Geometry: final body of the model. Coordinates: model frame, mm. A direction names the side the tool comes from. Give positions to 0.01 mm unless a question says otherwise; leave off trailing zeros. Loops run counter-clockwise (first coordinate to the right, second up) from the corner with the lowest first, then second, coordinate; pieces in that order, holes last. Notation, with made-up numbers: (5.5, 9) - (25.5, 9) arc R8 ccw to (25.5, 16) - close; hole circle Ø2 at (35, -18.5). An arc over 180 degrees is marked (long way). Use one line per item in the form item = value.
```python
from build123d import *

# Parameters (mm, degrees)
F1_DEPTH = 100
F2_T     = -2
F3_R     = 40
F4_DEPTH = 2
F5_R     = 4
F6_DEPTH = 2
F5_R_2   = 5
F7_DEPTH = 10
F8_SIZE2 = 3
F8_SIZE  = 0.6


with BuildPart() as f1:
    # F0 (on Front) → F1 (new body)
    with BuildSketch(Plane.XZ):
        Polygon((34.6410161514, -60), (69.2820323028, 0), (34.6410161514, 60), (-34.6410161514, 60), (-69.2820323028, 0), (-34.6410161514, -60), align=None)
    extrude(amount=F1_DEPTH)

    # F2
    f2_openings = [f1.faces().sort_by_distance(p)[0] for p in [
        (0, -100, 0),
    ]]
    offset(amount=F2_T, openings=f2_openings)

    # F3 (on face) → F4 (join)
    with BuildSketch(Plane.XZ.offset(100)):
        Polygon((-33.486315613, -58), (33.486315613, -58), (66.972631226, 0), (33.486315613, 58), (-33.486315613, 58), (-66.972631226, 0), align=None)
        Circle(F3_R, mode=Mode.SUBTRACT)
    extrude(amount=-F4_DEPTH)

    # F5 (on face) → F6 (cut, through all)
    with BuildSketch(Plane(origin=(0, 0, -60), x_dir=(1, 0, 0), z_dir=(0, 0, -1))):
        with Locations((0, 8.7902189698)):
            Circle(F5_R)
    extrude(amount=-F6_DEPTH, mode=Mode.SUBTRACT)

    # F5 (on face) → F7 (join)
    with BuildSketch(Plane(origin=(0, 0, -60), x_dir=(1, 0, 0), z_dir=(0, 0, -1))):
        with Locations((0, 8.7902189698)):
            Circle(F5_R_2)
        with Locations((0, 8.7902189698)):
            Circle(F5_R, mode=Mode.SUBTRACT)
    extrude(amount=F7_DEPTH)

    # F8
    f8_edges = [f1.edges().sort_by_distance(p)[0] for p in [
        (-5, -8.790219, -70),
    ]]
    f8_side = f1.faces().sort_by_distance((-4.858579, -8.790219, -70))[0]
    chamfer(f8_edges, length=F8_SIZE, length2=F8_SIZE2, reference=f8_side)


solid = f1.part
```
(1) Material intervals for L1, parallel to Z at x = -6, y = -77; L2, parallel to Y at x = 0, z = -66; L3, parallel to Z at x = 0, y = -99.1, sorted ascending. Write a range as from..to.
Solution:
L1 = -60..-58, 58..60
L2 = -13.79..-12.79, -4.79..-3.79
L3 = -60..-40, 40..60
(2) Cut plane A-A (x = 0). Return the cut outline in (y, z), plus the area to 3 significant figures.
Solution:
outline = (-100, -60) - (-13.79, -60) - (-13.79, -67) - (-13.19, -70) - (-12.79, -70) - (-12.79, -58) - (-98, -58) - (-98, -40) - (-100, -40) - close; (-100, 40) - (-98, 40) - (-98, 58) - (-2, 58) - (-2, -58) - (-4.79, -58) - (-4.79, -70) - (-4.39, -70) - (-3.79, -67) - (-3.79, -60) - (0, -60) - (0, 60) - (-100, 60) - close
area = 706 mm2
(3) Cut plane C-C (x = 51.5). Return the cut outline in (y, z), plus the area to 3 significant figures.
Solution:
outline = (-100, -30.8) - (0, -30.8) - (0, 30.8) - (-100, 30.8) - close; hole (-98, -26.8) - (-2, -26.8) - (-2, 26.8) - (-98, 26.8) - close
area = 1,010 mm2
(4) Access query for faces 1 (the face through (-8.67, -99.01, -39.05)), 2 (the face through (50, -49.3, -29.4)), 3 (the face through (-1.08, -3.91, -63.45)). Directions: +Z, -Z, +X, -X, +Y, -Y. A direction counts if a zero-diameter tool reaches every point of the face in a straight line with its end or side. Return the directions, or none.
Solution:
face_1 = -Y
face_2 = none
face_3 = -Z
(5) Cut plane D-D (z = -47.5). Return the cut outline in (x, y), plus the area to 3 significant figures.
Solution:
outline = (-41.86, -100) - (41.86, -100) - (41.86, 0) - (-41.86, 0) - close; hole (-39.55, -98) - (39.55, -98) - (39.55, -2) - (-39.55, -2) - close
area = 778 mm2
(6) Pull-direction query (Z, two-part tool) for faces 4 (the face through (0, -49, -58)), 5 (the face through (51.72, -49.3, -30.42)), 6 (the face through (-51.72, -49.3, 30.42)); classes: released by +Z, released by -Z, zero draft, split by the parting line, or undercut.
Solution:
face_4 = undercut
face_5 = released by -Z
face_6 = released by +Z
(7) Pin query (flat end, axial travel): P1, Ø2, axis at y = -70.5, z = 34, coming from the -X side; P2, Ø5, axis at y = -68.5, z = 34, coming from the +X side; P3, Ø4, axis at y = -70, z = -55, coming from the -X side. Return the tip coordinate at first contact, or that it passes through.
Solution:
P1 = -50.23
P2 = 51.1
P3 = -38.68
(8) Cut plane B-B (y = -84). Return the cut outline in (x, z).
Solution:
outline = (-69.28, 0) - (-34.64, -60) - (34.64, -60) - (69.28, 0) - (34.64, 60) - (-34.64, 60) - close; hole (-66.97, 0) - (-33.49, -58) - (33.49, -58) - (66.97, 0) - (33.49, 58) - (-33.49, 58) - close
